Design review of the part built by this model. Coordinates are the model's own, in mm. A direction names the side the tool comes from. Give positions to 0.01 mm unless a question says otherwise; leave off trailing zeros. Order: outer loops, then holes, each group sorted by start corner. A loop starts at its lowest first (then second) coordinate and runs counter-clockwise, first axis right, second up. Notation, with made-up numbers: M -19,-13 L 21,-13 A25 cw 21,13 Z; hole C -17.75,74 d1. An arc over 180 degrees is marked long. Answer as a JSON object with one key per item and string values.
from build123d import *

# Parameters (mm, degrees)
SKETCH1_W           = 40
SKETCH1_H           = 20
BOSS_EXTRUDE4_DEPTH = 35.32
SKETCH3_W           = 40
SKETCH3_H           = 93.52
BOSS_EXTRUDE5_DEPTH = 7
SKETCH4_R           = 12.5
CUT_EXTRUDE1_DEPTH  = 2.6
SKETCH5_R           = 6
CUT_EXTRUDE2_DEPTH  = 1.07
SKETCH6_R           = 2.5
CUT_EXTRUDE3_DEPTH  = 4
SKETCH7_R           = 1.25
CUT_EXTRUDE5_DEPTH  = 6
SKETCH9_R           = 2.7
CUT_EXTRUDE6_DEPTH  = 2
SKETCH10_R          = 1.5
CUT_EXTRUDE8_DEPTH  = 20
FILLET1_R           = 20
FILLET2_R           = 20
SKETCH11_W          = 45.672001295
SKETCH11_H          = 21.162412363
CUT_EXTRUDE9_DEPTH  = 5
CUT_EXTRUDE10_DEPTH = 10
FILLET5_R           = 10
FILLET6_R           = 10
FILLET7_R           = 10
FILLET8_R           = 10
FILLET9_R           = 2
FILLET10_R          = 2


with BuildPart() as part:
    # Sketch1 → Boss-Extrude4 (new body)
    with BuildSketch(Plane.XY):
        with Locations((20, -10)):
            Rectangle(SKETCH1_W, SKETCH1_H)
    extrude(amount=BOSS_EXTRUDE4_DEPTH)

    # Sketch3 → Boss-Extrude5 (add)
    with BuildSketch(Plane.XY.offset(35.32)):
        with Locations((20, 26.76)):
            Rectangle(SKETCH3_W, SKETCH3_H)
    extrude(amount=BOSS_EXTRUDE5_DEPTH)

    # Sketch4 → Cut-Extrude1 (cut)
    with BuildSketch(Plane.XY.offset(42.32)):
        with Locations((20, 58.46128741)):
            Circle(SKETCH4_R)
    extrude(amount=-CUT_EXTRUDE1_DEPTH, mode=Mode.SUBTRACT)

    # Sketch5 → Cut-Extrude2 (cut)
    with BuildSketch(Plane.XY.offset(39.72)):
        with Locations((20, 58.46128741)):
            Circle(SKETCH5_R)
    extrude(amount=-CUT_EXTRUDE2_DEPTH, mode=Mode.SUBTRACT)

    # Sketch6 → Cut-Extrude3 (cut)
    with BuildSketch(Plane.XY.offset(38.65)):
        with Locations((20, 58.46128741)):
            Circle(SKETCH6_R)
    extrude(amount=-CUT_EXTRUDE3_DEPTH, mode=Mode.SUBTRACT)

    # Sketch7 → Cut-Extrude5 (cut)
    with BuildSketch(Plane.XY.offset(39.72)):
        with Locations((27.794228634, 53.96128741)):
            Circle(SKETCH7_R)
        with Locations((12.205771366, 53.96128741)):
            Circle(SKETCH7_R)
        with Locations((20, 67.46128741)):
            Circle(SKETCH7_R)
    extrude(amount=-CUT_EXTRUDE5_DEPTH, mode=Mode.SUBTRACT)

    # Sketch9 → Cut-Extrude6 (cut)
    with BuildSketch(Plane(origin=(0, 0, 35.32), x_dir=(-1, 0, 0), z_dir=(0, 0, -1))):
        with Locations((-27.794228634, 53.96128741)):
            Circle(SKETCH9_R)
        with Locations((-12.205771366, 53.96128741)):
            Circle(SKETCH9_R)
        with Locations((-20, 67.46128741)):
            Circle(SKETCH9_R)
    extrude(amount=-CUT_EXTRUDE6_DEPTH, mode=Mode.SUBTRACT)

    # Sketch10 → Cut-Extrude8 (cut)
    with BuildSketch(Plane(origin=(0, 0, 0), x_dir=(-1, 0, 0), z_dir=(0, 0, -1))):
        with Locations((-30, -10)):
            Circle(SKETCH10_R)
        with Locations((-10, -10)):
            Circle(SKETCH10_R)
    extrude(amount=-CUT_EXTRUDE8_DEPTH, mode=Mode.SUBTRACT)

    # Fillet1
    fillet1_edges = [part.edges().sort_by_distance(p)[0] for p in [
        (20, 0, 35.32),
    ]]
    fillet(fillet1_edges, radius=FILLET1_R)

    # Fillet2
    fillet2_edges = [part.edges().sort_by_distance(p)[0] for p in [
        (20, -20, 42.32),
    ]]
    fillet(fillet2_edges, radius=FILLET2_R)

    # Sketch11 → Cut-Extrude9 (cut)
    with BuildSketch(Plane(origin=(0, 0, 0), x_dir=(-1, 0, 0), z_dir=(0, 0, -1))):
        with Locations((-18.602034722, -10.581206182)):
            Rectangle(SKETCH11_W, SKETCH11_H)
    extrude(amount=-CUT_EXTRUDE9_DEPTH, mode=Mode.SUBTRACT)

    # Sketch12 → Cut-Extrude10 (cut)
    with BuildSketch(Plane.XY.offset(42.32)):
        Polygon((0, 36.76), (8, 73.52), (0, 73.52), align=None)
        Polygon((32, 73.52), (40, 36.76), (40, 73.52), align=None)
    extrude(amount=-CUT_EXTRUDE10_DEPTH, mode=Mode.SUBTRACT)

    # Fillet5
    fillet5_edges = [part.edges().sort_by_distance(p)[0] for p in [
        (8, 73.52, 38.82),
    ]]
    fillet(fillet5_edges, radius=FILLET5_R)

    # Fillet6
    fillet6_edges = [part.edges().sort_by_distance(p)[0] for p in [
        (32, 73.52, 38.82),
    ]]
    fillet(fillet6_edges, radius=FILLET6_R)

    # Fillet7
    fillet7_edges = [part.edges().sort_by_distance(p)[0] for p in [
        (0, 36.76, 38.82),
    ]]
    fillet(fillet7_edges, radius=FILLET7_R)

    # Fillet8
    fillet8_edges = [part.edges().sort_by_distance(p)[0] for p in [
        (40, 36.76, 38.82),
    ]]
    fillet(fillet8_edges, radius=FILLET8_R)

    # Fillet9
    fillet9_edges = [part.edges().sort_by_distance(p)[0] for p in [
        (9.783440256, 71.306688481, 42.32),
        (36.742387874, 51.728727718, 42.32),
        (20, 73.52, 42.32),
        (30.216559744, 71.306688481, 42.32),
        (3.257612126, 51.728727718, 42.32),
        (0, 17.842224217, 42.32),
        (0.057343518, 36.753832409, 42.32),
        (39.942656482, 36.753832409, 42.32),
        (40, 17.842224217, 42.32),
        (40, -20, 13.66),
        (40, -14.142135624, 36.462135624),
        (0, -20, 13.66),
        (0, -14.142135624, 36.462135624),
    ]]
    fillet(fillet9_edges, radius=FILLET9_R)

    # Fillet10
    fillet10_edges = [part.edges().sort_by_distance(p)[0] for p in [
        (9.783440256, 71.306688481, 35.32),
        (36.742387874, 51.728727718, 35.32),
        (20, 73.52, 35.32),
        (30.216559744, 71.306688481, 35.32),
        (3.257612126, 51.728727718, 35.32),
        (0, 27.842224217, 35.32),
        (0.057343518, 36.753832409, 35.32),
        (39.942656482, 36.753832409, 35.32),
        (40, 27.842224217, 35.32),
        (0, 0, 10.16),
        (40, 0, 10.16),
        (0, 5.857864376, 29.462135624),
        (40, 5.857864376, 29.462135624),
    ]]
    fillet(fillet10_edges, radius=FILLET10_R)


solid = part.part
(1) Tool access review of faces 4 (the cylindrical face through (25.54, 56.16, 39.19)), 5 (the flat face through (20, 40, 35.32)), 6 (the cylindrical face through (39.4, -0.57, 10.09)): name each direction out of +Z, -Z, +X, -X, +Y, -Y from which nothing blocks a thin tool from reaching the whole face with its end or side.
Checked values:
{"face 4": "+Z", "face 5": "-Z, +X, -X, +Y", "face 6": "-Z, +X, +Y"}
(2) To check wall thickness, follow L1, parallel to Y at x = 20, z = 36.45; L2, parallel to Y at x = 10, z = 15; L3, parallel to Z at x = 3.5, y = 32. State the ranges of each line that lie inside material, in increasing order. Write a range as from..to.
Checked values:
{"L1": "y = -14.15..55.96, 60.96..64.76, 70.16..73.32", "L2": "y = -20..-11.5, -8.5..0", "L3": "z = 35.32..42.32"}
(3) We need section A-A (x = 20). Count the separate pieces of the cut face and the enclosed holes in it, plus the area to 3 significant figures.
Checked values:
{"separate pieces": "3", "enclosed holes": "0", "area": "1,150 mm^2"}
(4) We need section B-B (y = 27.5). Write out the cut boundary in (x, z), plus the area to 3 significant figures.
Checked values:
{"outline": "M 0,37.32 A2 ccw 2,35.32 L 38,35.32 A2 ccw 40,37.32 L 40,40.32 A2 ccw 38,42.32 L 2,42.32 A2 ccw 0,40.32 Z", "area": "277 mm^2"}
(5) Insertion check: pin 1 (1.5 mm diameter, centred on x = 20, y = 67.46, fed in from +Z); pin 2 (12 mm diameter, centred on x = 14.5, y = 43, fed in from -Z); pin 3 (4 mm diameter, centred on x = 12.21, y = 53.96, fed in from -Z); pin 4 (7.5 mm diameter, centred on x = 16.5, y = 62, fed in from +Z). Each pin has a flat end and moves straight along its axis. Give the tip position at first contact, or say it passes through.
Checked values:
{"pin 1": "passes through", "pin 2": "stops at z = 35.32", "pin 3": "stops at z = 37.32", "pin 4": "stops at z = 39.72"}
(6) Draft analysis for pull direction X (two halves, no side actions). For faces 1 (the flat face through (23, 59, 38.65)), 2 (the cylindrical face through (20.06, 72.95, 41.72)), 3 (the cylindrical face through (39.4, 27.73, 35.89)), state which applies: +X half, -X half, draft (parallel to the pull), parting line (faces both ways), or undercut.
Checked values:
{"face 1": "undercut", "face 2": "draft", "face 3": "+X half"}
